Here's how the part is built. I have some questions about the finished solid (model axes, mm). A direction names the side the tool comes from. Round coordinates to 2 decimals unless told otherwise and drop trailing zeros. Loops run counter-clockwise (first coordinate to the right, second up) from the corner with the lowest first, then second, coordinate; pieces in that order, holes last. Notation, with made-up numbers: (38.5, 11) - (90.5, 11) arc R19 cw to (90.5, 41) - close; hole circle Ø10 at (31, -0.5). An arc over 180 degrees is marked (long way). Answer as a JSON object with one key per item and string values. Group by question number.
1) I want a section at B-B, the plane z = -28. Please give me the cut outline in (x, y), then the cut area to 3 significant figures.
2) If we mould it in two halves opening along Z, with no side actions, what happens to faces 1 (the face through (78.076, -6, 32)), 2 (the face through (-63, -1.2, -12)), 3 (the face through (1, -1.2, -116)), 4 (the face through (1.48, 1.48, -33.31))? For each: pulls with the +Z half, pulls with the -Z half, needs draft (parallel to the pull), parting line crosses it, or undercut.
3) Will these pins go through, and if not, where does the flat tip stop? P1, Ø3.5, axis at x = 4, z = -118.5, coming from the -Y side; P2, Ø1.5, axis at y = -0.5, z = -9.5, coming from the -X side; P3, Ø6, axis at x = -5, y = -4.5, coming from the -Z side; P4, Ø9.5, axis at x = 3.08, z = -46, coming from the +Y side.
4) I want a section at C-C, the plane x = 54.5. Please give me the cut outline in (y, z), then the cut area to 3 significant figures.
5) I want a section at D-D, the plane z = -87. Please give me the cut outline in (x, y).
6) If I drill on line 1 along Y through (x, z) = (-6, -57); line 2 along X through (y, z) = (-5.75, 28); line 3 along Z through (x, y) = (-61, 2), over which ranges is the centre line in solid material (lowest first)? Write a range as [from, to].
7) I want a section at A-A, the plane z = 19. Please give me the cut outline in (x, y).
8) Which directions (+Z, -Z, +X, -X, +Y, -Y) give clear straight access to the entire face, cutting with the end or side of a thin tool? Please do faces 5 (the face through (-61.17, -4.71, -19.59)), 6 (the face through (-77, -5, 23)), 7 (the face through (-77, -2.1, 31)).
from build123d import *

# Parameters (mm, degrees)
BOSS_EXTRUDE1_DEPTH = 3
SKETCH2_W           = 13
SKETCH2_H           = 15
BOSS_EXTRUDE2_DEPTH = 2.8
SKETCH3_W           = 10.9
SKETCH3_H           = 7.8
SKETCH3_H_2         = 5.3
BOSS_EXTRUDE3_DEPTH = 15
SKETCH4_W           = 10.9
SKETCH4_H           = 2.5
BOSS_EXTRUDE4_DEPTH = 7.9
FILLET3_R           = 13
SKETCH5_R           = 5.6
SKETCH5_R_2         = 2.1
BOSS_EXTRUDE5_DEPTH = 5
CUT_EXTRUDE1_START  = -7.9
SKETCH6_R           = 2.1
CUT_EXTRUDE1_DEPTH  = 7.9
SKETCH7_R           = 3.7
CUT_EXTRUDE2_DEPTH  = 4.2
FILLET5_R           = 2
SKETCH8_R           = 5.6
SKETCH8_R_2         = 2.1
BOSS_EXTRUDE6_DEPTH = 2.5


with BuildPart() as part:
    # Sketch1 → Boss-Extrude1 (new body)
    with BuildSketch(Plane(origin=(0, 0, 0), x_dir=(1, 0, 0), z_dir=(0, 1, 0))):
        with BuildLine():
            Line((78.076457806, -38), (91.076457806, -38))
            Line((91.076457806, -38), (91.076457806, 130.104439919))
            Line((91.076457806, 130.104439919), (-84.923542194, 130.104439919))
            Line((-84.923542194, 130.104439919), (-84.923542194, 72.662298294))
            Line((-84.923542194, 72.662298294), (-84.923542194, 61.104439919))
            ThreePointArc((-84.923542194, 61.104439919), (-73.14747421, 32.674496882), (-84.923542194, 4.244553845))
            Line((-84.923542194, 4.244553845), (-84.923542194, 0))
            Line((-84.923542194, 0), (-84.923542194, -38))
            Line((-84.923542194, -38), (-71.923542194, -38))
            ThreePointArc((-71.923542194, -38), (3.076457806, 33.325120397), (78.076457806, -38))
        make_face()
    extrude(amount=BOSS_EXTRUDE1_DEPTH)

    # Sketch2 → Boss-Extrude2 (add)
    with BuildSketch(Plane.XY.offset(38)):
        with Locations((84.576457806, -4.5)):
            Rectangle(SKETCH2_W, SKETCH2_H)
        with Locations((-78.423542194, -4.5)):
            Rectangle(SKETCH2_W, SKETCH2_H)
    extrude(amount=BOSS_EXTRUDE2_DEPTH)

    # Sketch3 → Boss-Extrude3 (add)
    with BuildSketch(Plane(origin=(0, 0, 38), x_dir=(-1, 0, 0), z_dir=(0, 0, -1))):
        with Locations((-83.526457806, -6)):
            Rectangle(SKETCH3_W, SKETCH3_H)
        with Locations((77.373542194, -4.75)):
            Rectangle(SKETCH3_W, SKETCH3_H_2)
    extrude(amount=BOSS_EXTRUDE3_DEPTH)

    # Sketch4 → Boss-Extrude4 (add)
    with BuildSketch(Plane(origin=(0, 0, 38), x_dir=(-1, 0, 0), z_dir=(0, 0, -1))):
        with Locations((77.373542194, -8.65)):
            Rectangle(SKETCH4_W, SKETCH4_H)
    extrude(amount=BOSS_EXTRUDE4_DEPTH)

    # Fillet3
    fillet3_edges = [part.edges().sort_by_distance(p)[0] for p in [
        (-84.923542194, 1.5, -130.104439919),
        (91.076457806, 1.5, -130.104439919),
        (-84.923542194, 1.5, -4.244553845),
        (-84.923542194, 1.5, -61.104439919),
    ]]
    fillet(fillet3_edges, radius=FILLET3_R)

    # Sketch5 → Boss-Extrude5 (add)
    # profile 1 of 3: a face of its own
    with BuildSketch(Plane.XZ):
        with Locations(Location((3.076457806, -45.995120397, 0), (0, 0, 90))):
            Circle(SKETCH5_R)
        with Locations(Location((3.076457806, -45.995120397, 0), (0, 0, 270))):
            Circle(SKETCH5_R_2, mode=Mode.SUBTRACT)
    # profile 2 of 3: a face of its own
    with BuildSketch(Plane.XZ):
        with Locations(Location((-60.923542194, -13.995120397, 0), (0, 0, 90))):
            Circle(SKETCH5_R)
        with Locations(Location((-60.923542194, -13.995120397, 0), (0, 0, 270))):
            Circle(SKETCH5_R_2, mode=Mode.SUBTRACT)
    # profile 3 of 3: a face of its own
    with BuildSketch(Plane.XZ):
        with Locations(Location((3.076457806, -117.995120397, 0), (0, 0, 90))):
            Circle(SKETCH5_R)
        with Locations(Location((3.076457806, -117.995120397, 0), (0, 0, 270))):
            Circle(SKETCH5_R_2, mode=Mode.SUBTRACT)
    extrude(amount=BOSS_EXTRUDE5_DEPTH)

    # Sketch6 → Cut-Extrude1 (cut)
    with BuildSketch(Plane(origin=(0, 0, 0), x_dir=(-1, 0, 0), z_dir=(0, -1, 0)).offset(CUT_EXTRUDE1_START)):
        with Locations(Location((-3.076457806, 45.995120397, 0), (0, 0, 270))):
            Circle(SKETCH6_R)
        with Locations(Location((60.923542194, 13.995120397, 0), (0, 0, 270))):
            Circle(SKETCH6_R)
        with Locations(Location((-3.076457806, 117.995120397, 0), (0, 0, 270))):
            Circle(SKETCH6_R)
    extrude(amount=CUT_EXTRUDE1_DEPTH, mode=Mode.SUBTRACT)

    # Sketch7 → Cut-Extrude2 (cut)
    with BuildSketch(Plane(origin=(0, 3, 0), x_dir=(1, 0, 0), z_dir=(0, 1, 0))):
        with Locations(Location((3.076457806, 45.995120397, 0), (0, 0, 270))):
            Circle(SKETCH7_R)
        with Locations(Location((-60.923542194, 13.995120397, 0), (0, 0, 270))):
            Circle(SKETCH7_R)
        with Locations(Location((3.076457806, 117.995120397, 0), (0, 0, 270))):
            Circle(SKETCH7_R)
    extrude(amount=-CUT_EXTRUDE2_DEPTH, mode=Mode.SUBTRACT)

    # Fillet5
    fillet5_edges = [part.edges().sort_by_distance(p)[0] for p in [
        (3.076457806, 0, -51.595120397),
        (-60.923542194, 0, -19.595120397),
        (3.076457806, 0, -123.595120397),
    ]]
    fillet(fillet5_edges, radius=FILLET5_R)

    # Sketch8 → Boss-Extrude6 (add)
    # profile 1 of 2: a face of its own
    with BuildSketch(Plane.XZ.offset(5)):
        with Locations(Location((-60.923542194, -13.995120397, 0), (0, 0, 90))):
            Circle(SKETCH8_R)
        with Locations(Location((-60.923542194, -13.995120397, 0), (0, 0, 90))):
            Circle(SKETCH8_R_2, mode=Mode.SUBTRACT)
    # profile 2 of 2: a face of its own
    with BuildSketch(Plane.XZ.offset(5)):
        with Locations(Location((3.076457806, -117.995120397, 0), (0, 0, 90))):
            Circle(SKETCH8_R)
        with Locations(Location((3.076457806, -117.995120397, 0), (0, 0, 90))):
            Circle(SKETCH8_R_2, mode=Mode.SUBTRACT)
    extrude(amount=BOSS_EXTRUDE6_DEPTH)


solid = part.part
Outcome:
{
 "1": {"outline": "(-73.42, 0) - (-24.7, 0) - (-24.7, 3) - (-73.42, 3) - close; (30.85, 0) - (91.08, 0) - (91.08, 3) - (30.85, 3) - close", "area": "327 mm^2"},
 "2": {"face 1": "needs draft", "face 2": "undercut", "face 3": "undercut", "face 4": "pulls with the +Z half"},
 "3": {"P1": "y = -7.5", "P2": "x = -80.9", "P3": "z = -120.36", "P4": "y = 3"},
 "4": {"outline": "(0, -130.1) - (3, -130.1) - (3, -12.96) - (0, -12.96) - close", "area": "351 mm^2"},
 "5": {"outline": "(-84.92, 0) - (91.08, 0) - (91.08, 3) - (-84.92, 3) - close"},
 "6": {"line 1": "[0, 3]", "line 2": "[-82.82, -71.92], [78.08, 88.98]", "line 3": "[-130.1, -17.69], [-10.3, 2.61]"},
 "7": {"outline": "(-84.92, 0) - (-68.48, 0) - (-68.48, 3) - (-84.92, 3) - close; (74.64, 0) - (91.08, 0) - (91.08, 3) - (74.64, 3) - close"},
 "8": {"face 5": "-Y", "face 6": "-Z, +X, -X, -Y", "face 7": "-Z, +X, -X"}
}
